from build123d import *

# Parameters (mm, degrees)
SKETCH_1_R          = 1
EXTRUDE_1_DEPTH     = 3
SKETCH_2_W          = 16.007753667
SKETCH_2_H          = 50
EXTRUDE_2_DEPTH     = 80
CUT_EXTRUDE_1_DEPTH = 89.149011211
CUT_EXTRUDE_2_DEPTH = 81.960252593
EXTRUDE_3_DEPTH     = 3
CUT_EXTRUDE_3_DEPTH = 82.357621032
FILLET_1_R          = 0.5
FILLET_2_R          = 0.2


with BuildPart() as part:
    # 草图1 → 凸台-拉伸1 (new body)
    with BuildSketch(Plane(origin=(0, 0, 0), x_dir=(1, 0, 0), z_dir=(0, 1, 0))):
        with BuildLine():
            Line((-9.25, 25), (7.25, 25))
            ThreePointArc((7.25, 25), (8.664213562, 24.414213562), (9.25, 23))
            Line((9.25, 23), (9.25, -23))
            ThreePointArc((9.25, -23), (8.664213562, -24.414213562), (7.25, -25))
            Line((7.25, -25), (-9.25, -25))
            Line((-9.25, -25), (-9.25, 25))
        make_face()
        with Locations(Location((-1.25, 6, 0), (0, 0, 270))):
            Circle(SKETCH_1_R, mode=Mode.SUBTRACT)
        with Locations(Location((-1.25, -6, 0), (0, 0, 270))):
            Circle(SKETCH_1_R, mode=Mode.SUBTRACT)
        with Locations(Location((6.75, -6, 0), (0, 0, 270))):
            Circle(SKETCH_1_R, mode=Mode.SUBTRACT)
        with Locations(Location((6.75, 6, 0), (0, 0, 270))):
            Circle(SKETCH_1_R, mode=Mode.SUBTRACT)
    extrude(amount=EXTRUDE_1_DEPTH)

    # 草图2 → 凸台-拉伸2 (add)
    with BuildSketch(Plane(origin=(0, 3, 0), x_dir=(1, 0, 0), z_dir=(0, 1, 0))):
        with Locations((-1.246123166, 0)):
            Rectangle(SKETCH_2_W, SKETCH_2_H)
    extrude(amount=EXTRUDE_2_DEPTH)

    # 草图3 → 切除-拉伸1 (cut, through all)
    with BuildSketch(Plane(origin=(6.757753667, 0, 0), x_dir=(0, 0, -1), z_dir=(1, 0, 0))):
        Polygon((-25, 3), (-15, 15.5), (-3.181818182, 63), (1.818181818, 63), (25, 3), (32.784332669, 3), (32.784332669, 88.133626677), (-39.086773644, 88.133626677), (-39.086773644, 3), align=None)
        Polygon((-15, 3), (-8, 13), (0, 47), (17, 3), align=None)
    extrude(amount=-CUT_EXTRUDE_1_DEPTH, mode=Mode.SUBTRACT)

    # 草图4 → 切除-拉伸2 (cut, through all)
    with BuildSketch(Plane.XY.offset(25)):
        Polygon((6.757753667, 3), (6.757753667, 67.763295657), (-9.14963747, 67.763295657), align=None)
    extrude(amount=-CUT_EXTRUDE_2_DEPTH, mode=Mode.SUBTRACT)

    # 草图5 → 凸台-拉伸3 (add)
    with BuildSketch(Plane.ZY.offset(9.25)):
        Polygon((-1.818181818, 63), (-25, 3), (-25, 0), (25, 0), (25, 3), (15, 15.5), (3.181818182, 63), align=None)
        Polygon((0, 47), (-17, 3), (15, 3), (8, 13), align=None, mode=Mode.SUBTRACT)
    extrude(amount=EXTRUDE_3_DEPTH)

    # 草图6 → 切除-拉伸3 (cut, through all)
    with BuildSketch(Plane(origin=(0, 0, -25), x_dir=(-1, 0, 0), z_dir=(0, 0, -1))):
        Polygon((6.75, 0), (6.75, 13), (9.75, 45), (9.75, 64.870972757), (14.09361996, 64.870972757), (14.09361996, 0), align=None)
    extrude(amount=-CUT_EXTRUDE_3_DEPTH, mode=Mode.SUBTRACT)

    # 圆角1
    # the kernel refuses this fillet: 0.5 mm, written as the material it adds along each edge
    with BuildSketch(Plane(origin=(-6.75, 3, 15), x_dir=(0, 0, -1), z_dir=(1, 0, 0))) as fillet_1_piece_1_section:
        with BuildLine():
            CenterArc((FILLET_1_R * 1.92065556157, FILLET_1_R), FILLET_1_R, 145.007979801, 124.992020199)
            Line((FILLET_1_R * 1.10142364105, FILLET_1_R * 1.57346234436), (0, 0))
            Line((0, 0), (FILLET_1_R * 1.92065556157, 0))
        make_face()
    fillet_1_piece_1 = extrude(amount=15.908573119, mode=Mode.PRIVATE)
    fillet_1_piece_1 = split(fillet_1_piece_1, bisect_by=Plane(origin=(6.326718063, 4.754862629, 14.622728055), z_dir=(-0.9711342799096353, -0.23853345757858466, 0)), keep=Keep.TOP, mode=Mode.PRIVATE)
    add(fillet_1_piece_1)
    with BuildSketch(Plane(origin=(8.58076235, 3, -17), x_dir=(0, 0, 1), z_dir=(-1, 0, 0))) as fillet_1_piece_2_section:
        with BuildLine():
            CenterArc((FILLET_1_R * 1.45840694682, FILLET_1_R), FILLET_1_R, 158.875280854, 111.124719146)
            Line((FILLET_1_R * 0.525608812419, FILLET_1_R * 1.3603992792), (0, 0))
            Line((0, 0), (FILLET_1_R * 1.45840694682, 0))
        make_face()
    fillet_1_piece_2 = extrude(amount=15.33076235, mode=Mode.PRIVATE)
    fillet_1_piece_2 = split(fillet_1_piece_2, bisect_by=Plane(origin=(6.334852861, 4.721743663, -16.763347765), z_dir=(-0.9711342799096353, -0.23853345757858466, 0)), keep=Keep.TOP, mode=Mode.PRIVATE)
    add(fillet_1_piece_2)
    with BuildSketch(Plane(origin=(6.757753667, 3, 14.019874802), x_dir=(1, 0, 0), z_dir=(0, 0, 1))) as fillet_1_piece_3_section:
        with BuildLine():
            CenterArc((FILLET_1_R * 0.784100158108, FILLET_1_R), FILLET_1_R, 193.8, 76.2)
            Line((-FILLET_1_R * 0.187034121801, FILLET_1_R * 0.761466542421), (0, 0))
            Line((0, 0), (FILLET_1_R * 0.784100158108, 0))
        make_face()
    fillet_1_piece_3 = extrude(amount=10.980125198, mode=Mode.PRIVATE)
    fillet_1_piece_3 = split(fillet_1_piece_3, bisect_by=Plane(origin=(6.823819727, 0.737200979, 16.583959315), z_dir=(0, 0.5734623443633292, 0.8192319205190398)), keep=Keep.TOP, mode=Mode.PRIVATE)
    fillet_1_piece_3 = split(fillet_1_piece_3, bisect_by=Plane(origin=(6.823819727, 5.521194882, 22.983044095), z_dir=(0, -0.6246950475544246, -0.7808688094430302)), keep=Keep.TOP, mode=Mode.PRIVATE)
    add(fillet_1_piece_3)
    with BuildSketch(Plane(origin=(6.757753667, 3, -25), x_dir=(1, 0, 0), z_dir=(0, 0, 1))) as fillet_1_piece_4_section:
        with BuildLine():
            CenterArc((FILLET_1_R * 0.784100158108, FILLET_1_R), FILLET_1_R, 193.8, 76.2)
            Line((-FILLET_1_R * 0.187034121801, FILLET_1_R * 0.761466542421), (0, 0))
            Line((0, 0), (FILLET_1_R * 0.784100158108, 0))
        make_face()
    fillet_1_piece_4 = extrude(amount=8.980125198, mode=Mode.PRIVATE)
    fillet_1_piece_4 = split(fillet_1_piece_4, bisect_by=Plane(origin=(6.823760744, 4.428941995, -24.447908775), z_dir=(0, -0.36039927920216236, 0.9327981344055969)), keep=Keep.TOP, mode=Mode.PRIVATE)
    fillet_1_piece_4 = split(fillet_1_piece_4, bisect_by=Plane(origin=(6.823760744, 1.739503793, -17.487009898), z_dir=(0, 0.3603992792021622, -0.9327981344055969)), keep=Keep.TOP, mode=Mode.PRIVATE)
    add(fillet_1_piece_4)
    with BuildSketch(Plane(origin=(-6.75, 3, 15), x_dir=(0, 0, -1), z_dir=(1, 0, 0))) as fillet_1_piece_5a_section:
        with BuildLine():
            CenterArc((FILLET_1_R * 1.92065556157, FILLET_1_R), FILLET_1_R, 145.007979801, 124.992020199)
            Line((FILLET_1_R * 1.10142364105, FILLET_1_R * 1.57346234436), (0, 0))
            Line((0, 0), (FILLET_1_R * 1.92065556157, 0))
        make_face()
    fillet_1_piece_5a = extrude(amount=15.908573119, mode=Mode.PRIVATE)
    fillet_1_piece_5a = split(fillet_1_piece_5a, bisect_by=Plane(origin=(6.778509417, 2.915497721, 14.622764636), z_dir=(0.9711342799096353, 0.23853345757858466, 0)), keep=Keep.TOP, mode=Mode.PRIVATE)
    with BuildSketch(Plane(origin=(6.757753667, 3, 14.019874802), x_dir=(1, 0, 0), z_dir=(0, 0, 1))) as fillet_1_piece_5b_section:
        with BuildLine():
            CenterArc((FILLET_1_R * 0.784100158108, FILLET_1_R), FILLET_1_R, 193.8, 76.2)
            Line((-FILLET_1_R * 0.187034121801, FILLET_1_R * 0.761466542421), (0, 0))
            Line((0, 0), (FILLET_1_R * 0.784100158108, 0))
        make_face()
    fillet_1_piece_5b = extrude(amount=10.980125198, mode=Mode.PRIVATE)
    fillet_1_piece_5b = split(fillet_1_piece_5b, bisect_by=Plane(origin=(6.828403151, 3.296038352, 14.792773154), z_dir=(0, -0.5734623443633292, -0.8192319205190398)), keep=Keep.TOP, mode=Mode.PRIVATE)
    fillet_1_piece_5 = fillet_1_piece_5a & fillet_1_piece_5b
    add(fillet_1_piece_5)
    with BuildSketch(Plane(origin=(6.757753667, 3, -25), x_dir=(1, 0, 0), z_dir=(0, 0, 1))) as fillet_1_piece_6a_section:
        with BuildLine():
            CenterArc((FILLET_1_R * 0.784100158108, FILLET_1_R), FILLET_1_R, 193.8, 76.2)
            Line((-FILLET_1_R * 0.187034121801, FILLET_1_R * 0.761466542421), (0, 0))
            Line((0, 0), (FILLET_1_R * 0.784100158108, 0))
        make_face()
    fillet_1_piece_6a = extrude(amount=8.980125198, mode=Mode.PRIVATE)
    fillet_1_piece_6a = split(fillet_1_piece_6a, bisect_by=Plane(origin=(6.826253209, 3.240744299, -16.906985157), z_dir=(0, -0.3603992792021622, 0.9327981344055969)), keep=Keep.TOP, mode=Mode.PRIVATE)
    with BuildSketch(Plane(origin=(8.58076235, 3, -17), x_dir=(0, 0, 1), z_dir=(-1, 0, 0))) as fillet_1_piece_6b_section:
        with BuildLine():
            CenterArc((FILLET_1_R * 1.45840694682, FILLET_1_R), FILLET_1_R, 158.875280854, 111.124719146)
            Line((FILLET_1_R * 0.525608812419, FILLET_1_R * 1.3603992792), (0, 0))
            Line((0, 0), (FILLET_1_R * 1.45840694682, 0))
        make_face()
    fillet_1_piece_6b = extrude(amount=15.33076235, mode=Mode.PRIVATE)
    fillet_1_piece_6b = split(fillet_1_piece_6b, bisect_by=Plane(origin=(6.770254608, 2.949105284, -16.764105763), z_dir=(0.9711342799096353, 0.23853345757858466, 0)), keep=Keep.TOP, mode=Mode.PRIVATE)
    fillet_1_piece_6 = fillet_1_piece_6a & fillet_1_piece_6b
    add(fillet_1_piece_6)

    # 圆角2
    fillet_2_edges = [part.edges().sort_by_distance(p)[0] for p in [
        (-6.899841453, 47, 0),
    ]]
    fillet(fillet_2_edges, radius=FILLET_2_R)


solid = part.part
Geometry check sheet. Reference: the model listing, model coordinates, mm. A direction names the side the tool comes from. Give positions to 0.01 mm unless a question says otherwise; leave off trailing zeros. Loops run counter-clockwise (first coordinate to the right, second up) from the corner with the lowest first, then second, coordinate; pieces in that order, holes last. Notation, with made-up numbers: M 9,3 L 25,3 A21 cw 25,26 Z; hole C 23,27.25 d6. An arc over 180 degrees is marked long. Answer as a JSON object with one key per item and string values. Group by question number.
Item 1: Sectioned sample at D-D on y = 7. Record the boundary of the cut face in (x, z).
Item 2: Mould release check, pull along Y, two halves, no side actions. Record for faces 1 (the flat face through (-8.23, 28.78, 8.62)), 2 (the flat face through (-1.59, 9.34, 19.93)), 3 (the flat face through (1, 3, 0)), 4 (the flat face through (0, 8.33, 11.27)): pulls with the +Y half, pulls with the -Y half, needs draft (parallel to the pull), parting line crosses it, or undercut.
Item 3: Sectioned sample at B-B on y = 24. Record the boundary of the cut face in (x, z).
Item 4: Gauge pin test, flat ends, axial feed: pin 1 (14.5 mm diameter, centred on y = 8, z = -1, fed in from -X); pin 2 (1 mm diameter, centred on x = -6.5, y = 21.5, fed in from -Z); pin 3 (10 mm diameter, centred on x = 7, y = 12, fed in from -Z). Record the tip position at first contact, or that the pin passes through.
Item 5: Access from +Z, -Z, +X, -X, +Y, -Y to the whole of each face (thin tool, end or side, straight path). Record for faces 5 (the flat face through (-9.75, 52, -1)), 6 (the flat face through (-4.19, 29.45, 4.13)), 7 (the cylindrical face through (-1.86, 1.48, -6.79)), 8 (the cylindrical face through (7.426, 1.479, -6.737)), 9 (the flat face through (-6.75, 2, 0)).
Item 6: Sectioned sample at C-C on z = 6. Record the boundary of the cut face in (x, y).
Item 7: Material ranges on L1, parallel to X at y = 2.35, z = -6; L2, parallel to Z at x = 6.75, y = 1.25; L3, parallel to Y at x = 7, z = 12, recorded low to high.
Item 8: Sectioned sample at A-A on z = -14. Record the boundary of the cut face in (x, y), plus the area to 3 significant figures.
Findings below:
{
 "1": {"outline": "M -6.75,-23.45 L 5.78,-23.45 L 5.78,-15.45 L -6.75,-15.45 Z; M -6.75,12.2 L 5.78,12.2 L 5.78,21.8 L -6.75,21.8 Z"},
 "2": {"face 1": "pulls with the -Y half", "face 2": "pulls with the +Y half", "face 3": "undercut", "face 4": "undercut"},
 "3": {"outline": "M -7.78,-16.89 L 1.6,-16.89 L 1.6,-8.89 L -7.78,-8.89 Z; M -7.78,5.41 L 1.6,5.41 L 1.6,12.89 L -7.78,12.89 Z"},
 "4": {"pin 1": "x = -6.75", "pin 2": "z = -18.05", "pin 3": "z = -23.39"},
 "5": {"face 5": "+Z, -Z, -X, +Y, -Y", "face 6": "+X, -X", "face 7": "-Y", "face 8": "+Y, -Y", "face 9": "+Z, -Z, -X, -Y"},
 "6": {"outline": "M -9.75,45 L -7.55,21.5 L 2.21,21.5 L -5.2,51.67 L -9.75,51.67 Z; M -6.75,0 L -2.25,0 L -2.25,3 L -6.75,3 Z; M -0.25,0 L 5.75,0 L 5.75,3 L -0.25,3 Z; M 7.75,0 L 9.25,0 L 9.25,3 L 7.75,3 Z"},
 "7": {"L1": "-6.75 to -2.25, -0.25 to 5.75, 7.75 to 9.25", "L2": "-25 to -7, -5 to 5, 7 to 25", "L3": "0 to 3"},
 "8": {"outline": "M -8.48,31.47 L -6.75,13 L -6.75,10.76 L 4.85,10.76 L -0.24,31.47 Z; M -6.75,0 L 9.25,0 L 9.25,3 L -6.75,3 Z", "area": "252 mm2"}
}
